```python
from build123d import *

# Parameters (mm, degrees)
SKETCH1_W           = 600
SKETCH1_H           = 132
BOSS_EXTRUDE1_DEPTH = 18
SKETCH3_R           = 5
CUT_EXTRUDE2_DEPTH  = 584
SKETCH4_W           = 18
SKETCH4_H           = 50
CUT_EXTRUDE4_DEPTH  = 615.612072774
SKETCH5_W           = 100
SKETCH5_H           = 18
CUT_EXTRUDE5_DEPTH  = 615.612072774


with BuildPart() as part:
    # Sketch1 → Boss-Extrude1 (new body)
    with BuildSketch(Plane(origin=(0, 0, 0), x_dir=(0, 0, -1), z_dir=(1, 0, 0))):
        with Locations((300, -66)):
            Rectangle(SKETCH1_W, SKETCH1_H)
    extrude(amount=BOSS_EXTRUDE1_DEPTH)

    # Sketch3 → Cut-Extrude2 (cut)
    with BuildSketch(Plane(origin=(18, 0, 0), x_dir=(0, 0, -1), z_dir=(1, 0, 0))):
        with Locations((300, -66)):
            Circle(SKETCH3_R)
    extrude(amount=-CUT_EXTRUDE2_DEPTH, mode=Mode.SUBTRACT)

    # Sketch4 → Cut-Extrude4 (cut, through all)
    with BuildSketch(Plane(origin=(18, 0, 0), x_dir=(0, 0, -1), z_dir=(1, 0, 0))):
        with Locations((585, -66)):
            Rectangle(SKETCH4_W, SKETCH4_H)
        with Locations((15, -66)):
            Rectangle(SKETCH4_W, SKETCH4_H)
    extrude(amount=-CUT_EXTRUDE4_DEPTH, mode=Mode.SUBTRACT)

    # Sketch5 → Cut-Extrude5 (cut, through all)
    with BuildSketch(Plane(origin=(18, 0, 0), x_dir=(0, 0, -1), z_dir=(1, 0, 0))):
        with Locations((300, -117)):
            Rectangle(SKETCH5_W, SKETCH5_H)
    extrude(amount=-CUT_EXTRUDE5_DEPTH, mode=Mode.SUBTRACT)


solid = part.part
```
Could you check a few things on this model? Use its own coordinates, in mm. A direction names the side the tool comes from. Round coordinates to 2 decimals unless told otherwise and drop trailing zeros. Write each loop counter-clockwise with the first axis right and the second up, starting at its lowest first coordinate (ties: lowest second). Pieces come first, ordered by that corner, then holes.
(1) Suppose I cut it at B-B on z = -300. Write out the boundary of the cut face in (x, y).
Findings below:
outline: (0, -132) - (18, -132) - (18, -126) - (0, -126) - close; (0, -108) - (18, -108) - (18, -71) - (0, -71) - close; (0, -61) - (18, -61) - (18, 0) - (0, 0) - close
(2) If I drill on probe 1 along Y at (x, z) = (6.5, -300); probe 2 along Z at (x, y) = (12.5, -59.5); probe 3 along Y at (x, z) = (8.75, -290), over which ranges is the centre line in solid material (lowest first)?
Findings below:
probe 1: y = -132 to -126, -108 to -71, -61 to 0
probe 2: z = -600 to -594, -576 to -24, -6 to 0
probe 3: y = -132 to -126, -108 to 0
(3) Suppose I cut it at C-C on x = 5. Write out the boundary of the cut face in (y, z).
Findings below:
outline: (-132, -600) - (0, -600) - (0, 0) - (-132, 0) - close; hole (-126, -350) - (-108, -350) - (-108, -250) - (-126, -250) - close; hole (-91, -594) - (-41, -594) - (-41, -576) - (-91, -576) - close; hole (-91, -24) - (-41, -24) - (-41, -6) - (-91, -6) - close; hole circle Ø10 at (-66, -300)
(4) Thinking about a two-plate mould opening in Y: for faces 3 (the face through (9, 0, -296)), 4 (the face through (9, -41, -15)), 5 (the face through (0, -50, -296)), which applies, +Y half, -Y half, draft (parallel to the pull), parting line (faces both ways), or undercut?
Findings below:
face 3: +Y half
face 4: undercut
face 5: draft
(5) For pin 1 (9 mm diameter, centred on y = -66, z = -300, fed in from +X), with a flat end and sliding along its axis, tell me the tip position at first contact or that it passes through.
Findings below:
pin 1: passes through
(6) Suppose I cut it at A-A on y = -66. Write out the boundary of the cut face in (x, z).
Findings below:
outline: (0, -600) - (18, -600) - (18, -594) - (0, -594) - close; (0, -576) - (18, -576) - (18, -305) - (0, -305) - close; (0, -295) - (18, -295) - (18, -24) - (0, -24) - close; (0, -6) - (18, -6) - (18, 0) - (0, 0) - close
(7) Which directions (+Z, -Z, +X, -X, +Y, -Y) give clear straight access to the entire face, cutting with the end or side of a thin tool? Please do faces 1 (the face through (9, -66, -24)), 2 (the face through (9, -67, 0)).
Findings below:
face 1: +X, -X
face 2: +Z, +X, -X, +Y, -Y
